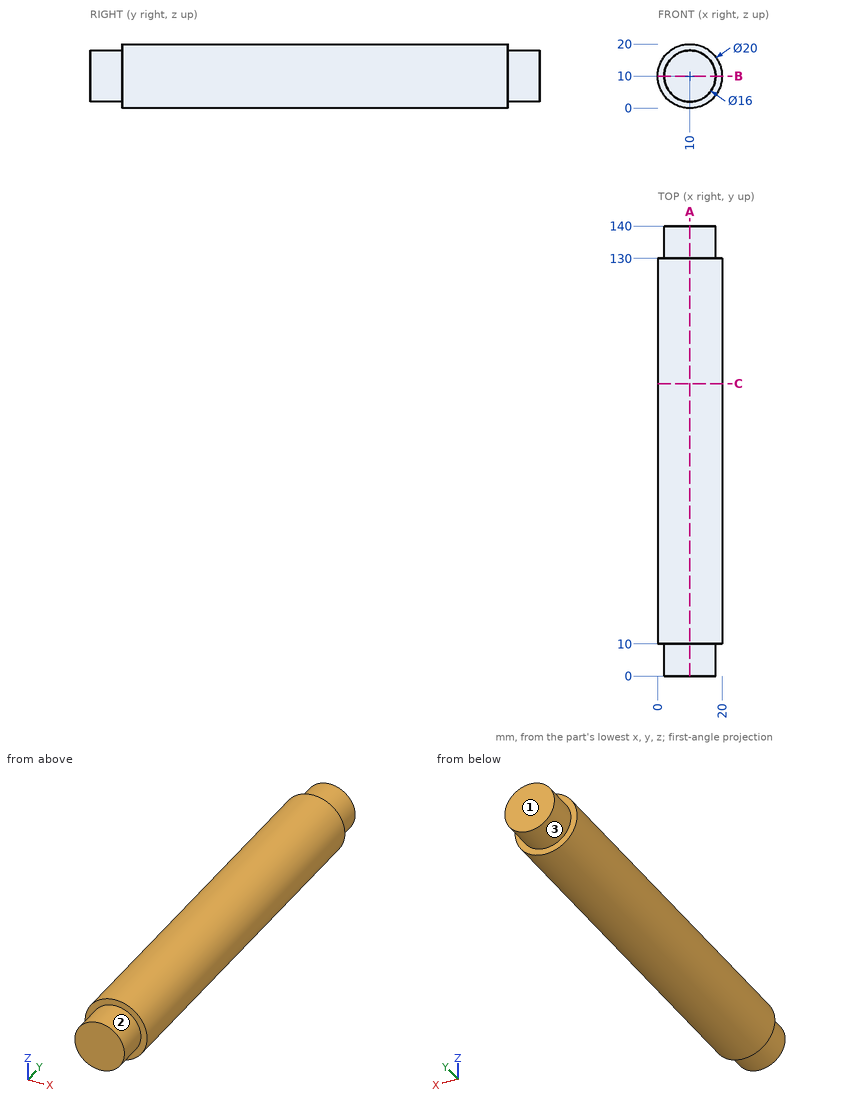
Here's the drawing with two shaded views (mm, measured from the low corner). I have some questions. A direction names the side the tool comes from. Give positions to 0.01 mm unless a question says otherwise; leave off trailing zeros. Loops run counter-clockwise (first coordinate to the right, second up) from the corner with the lowest first, then second, coordinate; pieces in that order, holes last. Notation, with made-up numbers: M 19.25,53.5 L 44.25,53.5 A26 ccw 44.25,78.5 Z; hole C 21.25,1 d2. An arc over 180 degrees is marked long. Use one line per item in the form item = value. Start each with the question number.
Q1. I need wall thicknesses on line 1 along Z through (x, y) = (16, 118.5); line 2 along Y through (x, z) = (6, 19); line 3 along Z through (x, y) = (9.75, 84.5). Which ranges of each line are inside material? Lowest first, please.
Q2. If we section it at A-A (x = 10): Write out the boundary of the cut face in (y, z).
Q3. If we section it at B-B (z = 10): Write out the boundary of the cut face in (x, y), then the cut area to 3 significant figures.
Q4. Which directions (+Z, -Z, +X, -X, +Y, -Y) give clear straight access to the entire face, cutting with the end or side of a thin tool? Please do the marked faces 1, 2 and 3.
Q5. Will these pins go through, and if not, where does the flat tip stop? pin 1 Ø3 at (x, y) = (17, 51) entering from -Z; pin 2 Ø4 at (x, y) = (16.5, 109.5) entering from +Z.
Q6. If we section it at C-C (y = 91): Write out the boundary of the cut face in (x, z).
Taken from the geometry:
q1.line_1 = 2 to 18
q1.line_2 = 10 to 130
q1.line_3 = 0 to 20
q2.outline = M 0,2 L 10,2 L 10,0 L 130,0 L 130,2 L 140,2 L 140,18 L 130,18 L 130,20 L 10,20 L 10,18 L 0,18 Z
q3.outline = M 0,10 L 2,10 L 2,0 L 18,0 L 18,10 L 20,10 L 20,130 L 18,130 L 18,140 L 2,140 L 2,130 L 0,130 Z
q3.area = 2,720 mm^2
q4.face_1 = +Z, -Z, +X, -X, +Y
q4.face_2 = -Y
q4.face_3 = +Y
q5.pin_1 = 1.65
q5.pin_2 = 18.93
q6.outline = C 10,10 d20
